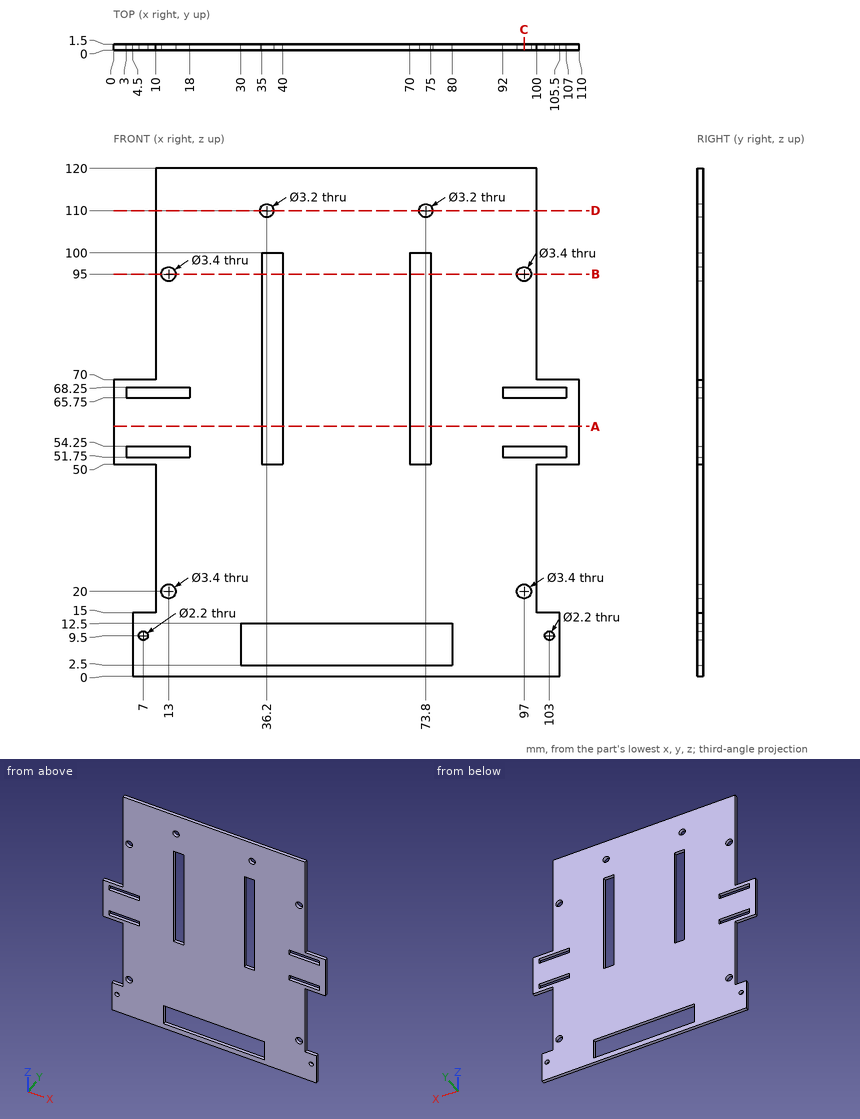
Input: dimensioned drawing with shaded views. Units: mm. Origin: part minimum x, y, z. Coordinates: 2 decimals unless noted, no trailing zeros. Loops run counter-clockwise (first coordinate to the right, second up) from the corner with the lowest first, then second, coordinate; pieces in that order, holes last.
Q1. Section D-D, the plane z = 110. Return the cut outline in (x, y).
Results are:
outline: (10, 0) - (34.6, 0) - (34.6, 1.5) - (10, 1.5) - close; (37.8, 0) - (72.2, 0) - (72.2, 1.5) - (37.8, 1.5) - close; (75.4, 0) - (100, 0) - (100, 1.5) - (75.4, 1.5) - close
Q2. Contact query for flat-ended pins moving along their axis: pin 1 (4 mm diameter, centred on x = 13, z = 20, fed in from -Y); pin 2 (0.8 mm diameter, centred on y = 0.5, z = 6, fed in from -X). Output: stop coordinate, or through.
Results are:
pin 1: stops at y = 0
pin 2: stops at x = 4.5
Q3. Section C-C, the plane x = 97. Return the cut outline in (y, z), and give its area (3 significant figures).
Results are:
outline: (0, 0) - (1.5, 0) - (1.5, 18.3) - (0, 18.3) - close; (0, 21.7) - (1.5, 21.7) - (1.5, 51.75) - (0, 51.75) - close; (0, 54.25) - (1.5, 54.25) - (1.5, 65.75) - (0, 65.75) - close; (0, 68.25) - (1.5, 68.25) - (1.5, 93.3) - (0, 93.3) - close; (0, 96.7) - (1.5, 96.7) - (1.5, 120) - (0, 120) - close
area: 162 mm2
Q4. Line query: line 1 along X through (y, z) = (0.2, 64); line 2 along X through (y, z) = (1.1, 90); line 3 along X through (y, z) = (0.65, 95). Output: solid intervals per line, ascending.
Results are:
line 1: x = 0 to 35, 40 to 70, 75 to 110
line 2: x = 10 to 35, 40 to 70, 75 to 100
line 3: x = 10 to 11.3, 14.7 to 35, 40 to 70, 75 to 95.3, 98.7 to 100
Q5. Section B-B, the plane z = 95. Return the cut outline in (x, y).
Results are:
outline: (10, 0) - (11.3, 0) - (11.3, 1.5) - (10, 1.5) - close; (14.7, 0) - (35, 0) - (35, 1.5) - (14.7, 1.5) - close; (40, 0) - (70, 0) - (70, 1.5) - (40, 1.5) - close; (75, 0) - (95.3, 0) - (95.3, 1.5) - (75, 1.5) - close; (98.7, 0) - (100, 0) - (100, 1.5) - (98.7, 1.5) - close
Q6. Section A-A, the plane z = 59. Return the cut outline in (x, y).
Results are:
outline: (0, 0) - (35, 0) - (35, 1.5) - (0, 1.5) - close; (40, 0) - (70, 0) - (70, 1.5) - (40, 1.5) - close; (75, 0) - (110, 0) - (110, 1.5) - (75, 1.5) - close
